Work out the finished part from the listing and answer in its coordinate system (mm). Face numbers are marked on the shaded views. A direction names the side the tool comes from. Coordinates: 2 decimals unless noted, no trailing zeros. Write each loop counter-clockwise with the first axis right and the second up, starting at its lowest first coordinate (ties: lowest second). Pieces come first, ordered by that corner, then holes. Notation, with made-up numbers: M 28,-11.75 L 47,-11.75 A18 cw 47,22.25 Z; hole C -16.75,26.5 d2. An arc over 180 degrees is marked long. Answer as CSV lines item,"result". Start each with the question number.
(1) Flat-ended cylindrical pins translate along their axes: P1, Ø14.5, axis at x = 38, z = -6, coming from the +Y side; P2, Ø6, axis at y = 24.5, z = 3.5, coming from the +X side. Find the tip coordinate at first contact, or state that the pin passes through.
(2) For the marked faces 1 and 2, determine the directions among +Z, -Z, +X, -X, +Y, -Y from which every point of the face is accessible in a straight line to the end or side of a thin tool.
(3) A cutting plane is placed at A-A on x = 42. Give the vertices of the cut face in (y, z).
(4) Find the intervals of material crossed by L1, parallel to X at y = 39, z = -6, in increasing order. Write a range as [from, to].
(5) A cutting plane is placed at B-B on z = -17.5. Give the vertices of the cut face in (x, y).
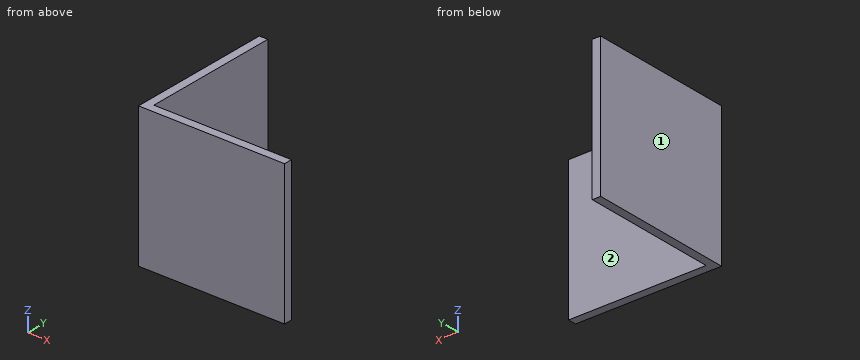
from build123d import *

# Parameters (mm, degrees)
BOSS_EXTRUDE1_DEPTH = 25.05


with BuildPart() as part:
    # Sketch1 → Boss-Extrude1 (new, symmetric)
    with BuildSketch(Plane.XY):
        Polygon((0, 0), (0, 52), (3, 52), (3, 3), (52, 3), (52, 0), align=None)
    boss_extrude1 = extrude(amount=BOSS_EXTRUDE1_DEPTH, both=True)


with BuildPart() as mirror1_1:
    # Mirror1: Boss-Extrude1 across plane
    add(boss_extrude1.mirror(Plane.XY))


with BuildPart() as part_1:
    add(part.part)

    # Mirror1 united with what the copies touc: union Mirror1_1
    add(mirror1_1.part)


solid = part_1.part
Here are the results:
1,P1,"stops at y = 3"
1,P2,"stops at x = 3"
2,face 1,"+Z, -Z, -X, +Y, -Y"
2,face 2,"+Z, -Z, +X, +Y"
3,outline,"M 0,-25.05 L 3,-25.05 L 3,25.05 L 0,25.05 Z"
4,L1,"x = [0, 3]"
5,outline,"M 0,0 L 52,0 L 52,3 L 3,3 L 3,52 L 0,52 Z"
